Read the model definition and answer for the solid it produces. Units are mm, in the model's axes. Coordinates: 2 decimals unless noted, no trailing zeros. Write each loop counter-clockwise with the first axis right and the second up, starting at its lowest first coordinate (ties: lowest second). Pieces come first, ordered by that corner, then holes. Notation, with made-up numbers: (24.25, -25) -> (65.25, -25) arc R11 ccw to (65.25, -15) -> close; hole circle Ø3 at (59, 70.5). An arc over 180 degrees is marked (long way). Return JSON: item names as keys, results as strings.
from build123d import *

# Parameters (mm, degrees)
SKETCH_1_R          = 47.5
SKETCH_1_R_2        = 35
EXTRUDE_1_DEPTH     = 5
CUT_EXTRUDE_1_REACH = 69.361
SKETCH_2_R          = 2.575


with BuildPart() as part:
    # 草图1 → 凸台-拉伸1 (new body)
    with BuildSketch(Plane(origin=(0, 0, 0), x_dir=(1, 0, 0), z_dir=(0, 1, 0))):
        with Locations(Location((0, 0, 0), (0, 0, 270))):
            Circle(SKETCH_1_R)
        with Locations(Location((0, 0, 0), (0, 0, 270))):
            Circle(SKETCH_1_R_2, mode=Mode.SUBTRACT)
    extrude(amount=EXTRUDE_1_DEPTH)

    # 草图2 → 切除-拉伸1 (cut, up to next)
    with BuildSketch(Plane(origin=(0, 5, 0), x_dir=(1, 0, 0), z_dir=(0, 1, 0)), mode=Mode.PRIVATE) as cut_extrude_1_sk1:
        with Locations(Location((0, 41, 0), (0, 0, 270))):
            Circle(SKETCH_2_R)
    cut_extrude_1_tool1 = extrude(cut_extrude_1_sk1.sketch, amount=-CUT_EXTRUDE_1_REACH, mode=Mode.PRIVATE) & part.part
    # 草图2 → 切除-拉伸1 (cut, up to next)
    with BuildSketch(Plane(origin=(0, 5, 0), x_dir=(1, 0, 0), z_dir=(0, 1, 0)), mode=Mode.PRIVATE) as cut_extrude_1_sk2:
        with Locations(Location((41, 0, 0), (0, 0, 270))):
            Circle(SKETCH_2_R)
    cut_extrude_1_tool2 = extrude(cut_extrude_1_sk2.sketch, amount=-CUT_EXTRUDE_1_REACH, mode=Mode.PRIVATE) & part.part
    # 草图2 → 切除-拉伸1 (cut, up to next)
    with BuildSketch(Plane(origin=(0, 5, 0), x_dir=(1, 0, 0), z_dir=(0, 1, 0)), mode=Mode.PRIVATE) as cut_extrude_1_sk3:
        with Locations(Location((0, -41, 0), (0, 0, 270))):
            Circle(SKETCH_2_R)
    cut_extrude_1_tool3 = extrude(cut_extrude_1_sk3.sketch, amount=-CUT_EXTRUDE_1_REACH, mode=Mode.PRIVATE) & part.part
    # 草图2 → 切除-拉伸1 (cut, up to next)
    with BuildSketch(Plane(origin=(0, 5, 0), x_dir=(1, 0, 0), z_dir=(0, 1, 0)), mode=Mode.PRIVATE) as cut_extrude_1_sk4:
        with Locations(Location((-41, 0, 0), (0, 0, 270))):
            Circle(SKETCH_2_R)
    cut_extrude_1_tool4 = extrude(cut_extrude_1_sk4.sketch, amount=-CUT_EXTRUDE_1_REACH, mode=Mode.PRIVATE) & part.part
    add(cut_extrude_1_tool1.solids().sort_by_distance((0, 5, -41))[0], mode=Mode.SUBTRACT)
    add(cut_extrude_1_tool2.solids().sort_by_distance((41, 5, 0))[0], mode=Mode.SUBTRACT)
    add(cut_extrude_1_tool3.solids().sort_by_distance((0, 5, 41))[0], mode=Mode.SUBTRACT)
    add(cut_extrude_1_tool4.solids().sort_by_distance((-41, 5, 0))[0], mode=Mode.SUBTRACT)


solid = part.part
1. The part is cut by section D-D (x = -23.5). Determine the outline of the cut face in (y, z), then the cut area to 3 significant figures.
Taken from the geometry:
{"outline": "(0, -41.28) -> (5, -41.28) -> (5, -25.94) -> (0, -25.94) -> close; (0, 25.94) -> (5, 25.94) -> (5, 41.28) -> (0, 41.28) -> close", "area": "153 mm2"}
2. The part is cut by section C-C (z = 41). Determine the outline of the cut face in (x, y) (3 decimals), then the cut area to 3 significant figures.
Taken from the geometry:
{"outline": "(-23.984, 0) -> (-2.575, 0) -> (-2.575, 5) -> (-23.984, 5) -> close; (2.575, 0) -> (23.984, 0) -> (23.984, 5) -> (2.575, 5) -> close", "area": "214 mm2"}
3. The part is cut by section B-B (x = 0). Determine the outline of the cut face in (y, z) (3 decimals), then the cut area to 3 significant figures.
Taken from the geometry:
{"outline": "(0, -47.5) -> (5, -47.5) -> (5, -43.575) -> (0, -43.575) -> close; (0, -38.425) -> (5, -38.425) -> (5, -35) -> (0, -35) -> close; (0, 35) -> (5, 35) -> (5, 38.425) -> (0, 38.425) -> close; (0, 43.575) -> (5, 43.575) -> (5, 47.5) -> (0, 47.5) -> close", "area": "73.5 mm2"}
4. The part is cut by section A-A (z = 0). Determine the outline of the cut face in (x, y) (3 decimals), then the cut area to 3 significant figures.
Taken from the geometry:
{"outline": "(-47.5, 0) -> (-43.575, 0) -> (-43.575, 5) -> (-47.5, 5) -> close; (-38.425, 0) -> (-35, 0) -> (-35, 5) -> (-38.425, 5) -> close; (35, 0) -> (38.425, 0) -> (38.425, 5) -> (35, 5) -> close; (43.575, 0) -> (47.5, 0) -> (47.5, 5) -> (43.575, 5) -> close", "area": "73.5 mm2"}
5. Consider L1, parallel to X at y = 2.8, z = 0 (3 decimals); L2, parallel to X at y = 4.35, z = -23; L3, parallel to X at y = 1.4, z = -7. Determine where each line is inside the solid, lowest interval first.
Taken from the geometry:
{"L1": "x = -47.5 to -43.575, -38.425 to -35, 35 to 38.425, 43.575 to 47.5", "L2": "x = -41.56 to -26.38, 26.38 to 41.56", "L3": "x = -46.98 to -34.29, 34.29 to 46.98"}
6. For a pull along Z with two mould halves and no side action, classify faces 1 (the face through (-3.3, 5, -35.4)), 2 (the face through (38.716, 2.535, 1.188)), 3 (the face through (-46.37, 2.46, -10.3)) as +Z half, -Z half, draft (parallel to the pull), parting line (faces both ways), or undercut.
Taken from the geometry:
{"face 1": "draft", "face 2": "undercut", "face 3": "parting line"}
7. Flat-ended cylindrical pins translate along their axes: pin 1 Ø1 at (x, y) = (-1, 3.5) entering from +Z; pin 2 Ø3 at (x, z) = (-41, 0) entering from +Y; pin 3 Ø6 at (x, z) = (0, -41) entering from +Y; pin 4 Ø3 at (y, z) = (1, 21) entering from -X. Find the tip coordinate at first contact, or state that the pin passes through.
Taken from the geometry:
{"pin 1": "stops at z = 47.5", "pin 2": "passes through", "pin 3": "stops at y = 5", "pin 4": "stops at x = -43.31"}
